Part model, mm, in its own coordinate system. Round coordinates to 2 decimals unless told otherwise and drop trailing zeros. Loops run counter-clockwise (first coordinate to the right, second up) from the corner with the lowest first, then second, coordinate; pieces in that order, holes last. Notation, with made-up numbers: (40, 63) -> (50, 63) arc R28 cw to (50, 91) -> close; hole circle Ø11 at (25.25, 26). An arc over 180 degrees is marked (long way). Answer as a JSON object with one key per item and string values. Group by question number.
from build123d import *

# Parameters (mm, degrees)
SKETCH1_W                    = 694
SKETCH1_H                    = 33
BASE_FLANGE1_DEPTH           = 2
EDGE_FLANGE1_STRIP_W         = 12
EDGE_FLANGE1_STRIP_H         = 2
EDGE_FLANGE1_STRIP_CUT_DEPTH = 694
EDGE_FLANGE1_DEPTH           = 694
EDGE_FLANGE2_DEPTH           = 634


# Sheet-metal steps are written as plain solids
with BuildPart() as part:
    # Sketch1 → Base-Flange1 (new body)
    with BuildSketch(Plane.XY):
        Rectangle(SKETCH1_W, SKETCH1_H)
    extrude(amount=BASE_FLANGE1_DEPTH)

    # Edge-Flange1 strip (across the edge) → Edge-Flange1 strip cut (cut)
    with BuildSketch(Plane(origin=(347, -16.5, 0), x_dir=(0, 1, 0), z_dir=(-1, 0, 0))):
        with Locations((-2, -1)):
            Rectangle(EDGE_FLANGE1_STRIP_W, EDGE_FLANGE1_STRIP_H)
    extrude(amount=EDGE_FLANGE1_STRIP_CUT_DEPTH, mode=Mode.SUBTRACT)

    # Edge-Flange1 section (across the edge) → Edge-Flange1 (add)
    with BuildSketch(Plane(origin=(347, -16.5, 0), x_dir=(0, 1, 0), z_dir=(-1, 0, 0))):
        with BuildLine():
            Line((0, 2), (0, 25))
            Line((0, 25), (2, 25))
            Line((2, 25), (2, 2))
            ThreePointArc((2, 2), (2.585786438, 0.585786438), (4, 0))
            Line((4, 0), (4, -2))
            ThreePointArc((4, -2), (1.171572875, -0.828427125), (0, 2))
        make_face()
    extrude(amount=EDGE_FLANGE1_DEPTH)

    # Edge-Flange2 section (across the edge) → Edge-Flange2 (add)
    with BuildSketch(Plane(origin=(-317, 17.130597578, 0), x_dir=(0, -0.5735764363510416, -0.8191520442889949), z_dir=(1, 0, 0))):
        with BuildLine():
            Line((-2, 0.630597578), (-2, 19.369402422))
            Line((-2, 19.369402422), (0, 19.369402422))
            Line((0, 19.369402422), (0, 0.630597578))
            ThreePointArc((0, 0.630597578), (0.092566099, 0.029185979), (0.361695911, -0.516555295))
            Line((0.361695911, -0.516555295), (-1.276608177, -1.663708168))
            ThreePointArc((-1.276608177, -1.663708168), (-1.814867803, -0.57222562), (-2, 0.630597578))
        make_face()
    extrude(amount=EDGE_FLANGE2_DEPTH)


solid = part.part
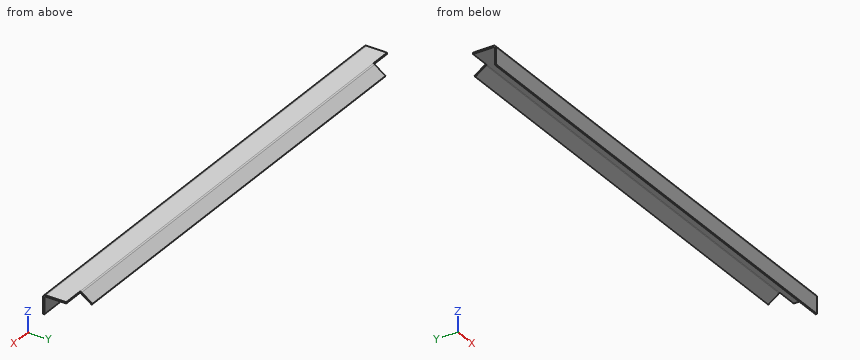
Item 1: Drill centre lines: line 1 (Z direction, x = -51.5, y = 8); line 2 (Y direction, x = -108.5, z = -21.5); line 3 (Y direction, x = 132.5, z = -3). Where is each one in solid material? Low to high.
Item 2: Band-saw the part on C-C, the plane y = 5.5. List the corners of the cut face in (x, z).
Item 3: Band-saw the part on B-B, the plane z = -17.25. List the corners of the cut face in (x, y).
Item 4: Drop flat-ended pins along their axis: pin 1 Ø8 at (x, y) = (-111.5, 1.5) entering from -Z; pin 2 Ø1.6 at (x, z) = (337.5, 0.5) entering from +Y; pin 3 Ø14.5 at (y, z) = (24.5, -4.5) entering from +X; pin 4 Ø10 at (y, z) = (9, -9) entering from -X. Give the stop position or say it passes through.
Item 5: Band-saw the part on A-A, the plane x = 52. List the corners of the cut face in (y, z), plus the area to 3 significant figures.
Entries:
{
 "1": {"line 1": "0 to 2", "line 2": "-16.5 to -14.5", "line 3": "-16.5 to -14.5, 21.42 to 24.9"},
 "2": {"outline": "(-347, 0) -> (347, 0) -> (347, 2) -> (-347, 2) -> close"},
 "3": {"outline": "(-347, -16.5) -> (347, -16.5) -> (347, -14.5) -> (-347, -14.5) -> close"},
 "4": {"pin 1": "z = 0", "pin 2": "y = 16.5", "pin 3": "x = 317", "pin 4": "through"},
 "5": {"outline": "(-16.5, -25) -> (-14.5, -25) -> (-14.5, -2) arc R2 cw to (-12.5, 0) -> (16.5, 0) arc R2 cw to (17.65, -0.36) -> (33, -11.11) -> (34.14, -9.47) -> (18.79, 1.28) arc R4 ccw to (16.5, 2) -> (-12.5, 2) arc R4 ccw to (-16.5, -2) -> close", "area": "155 mm²"}
}
